from build123d import *

# Parameters (mm, degrees)
F0_W          = 12.7
F0_H          = 12.7
F1_DEPTH      = 12.7
F2_R          = 6.35
F3_DEPTH      = 12.7
F4_W          = 12.7
F4_H          = 12.7
F5_DEPTH      = 12.7
F7_DEPTH      = 6.351
F7_DEPTH_BACK = 6.351
F9_DEPTH      = 6.351
F9_DEPTH_BACK = 6.351


with BuildPart() as f1:
    # F0 (on Top) → F1 (new body)
    with BuildSketch(Plane.XY):
        Rectangle(F0_W, F0_H)
    extrude(amount=F1_DEPTH)

    # F2 (on face) → F3 (join)
    with BuildSketch(Plane.XY.offset(12.7)):
        Circle(F2_R)
    extrude(amount=F3_DEPTH)

    # F4 (on face) → F5 (join)
    with BuildSketch(Plane.XY.offset(25.4)):
        Rectangle(F4_W, F4_H)
    extrude(amount=F5_DEPTH)

    # F6 (on Front) → F7 (cut, two sides)
    with BuildSketch(Plane.XZ) as f7_sk:
        Polygon((-4.445, 25.4), (0, 38.1), (-6.35, 38.1), (-6.35, 25.4), align=None)
        Polygon((4.445, 25.4), (6.35, 25.4), (6.35, 38.1), (0, 38.1), align=None)
    extrude(amount=-F7_DEPTH, mode=Mode.SUBTRACT)
    extrude(f7_sk.sketch, amount=F7_DEPTH_BACK, mode=Mode.SUBTRACT)

    # F8 (on Right) → F9 (cut, two sides)
    with BuildSketch(Plane.YZ) as f9_sk:
        Polygon((1.4e-09, 38.1), (-6.35, 38.1), (-6.35, 25.4), (-4.4449999986, 25.4), align=None)
        Polygon((6.35, 38.1), (1.4e-09, 38.1), (4.4450000014, 25.4), (6.35, 25.4), align=None)
    extrude(amount=-F9_DEPTH, mode=Mode.SUBTRACT)
    extrude(f9_sk.sketch, amount=F9_DEPTH_BACK, mode=Mode.SUBTRACT)


solid = f1.part
Verification items for the finished model (mm, model axes). A direction names the side the tool comes from. Give positions to 0.01 mm unless a question says otherwise; leave off trailing zeros. Loops run counter-clockwise (first coordinate to the right, second up) from the corner with the lowest first, then second, coordinate; pieces in that order, holes last.
1) Sectioned sample at A-A, the plane y = -2.5. Enter the section's corners in (x, z) (3 decimals).
2) Sectioned sample at D-D, the plane z = 29. Enter the section's corners in (x, y) (3 decimals), then the cut area to 3 significant figures.
3) Sectioned sample at C-C, the plane z = 33.5. Enter the section's corners in (x, y), then the cut area to 3 significant figures.
4) Thickness scan on line 1 along Z through (x, y) = (-4.25, 6); line 2 along Z through (x, y) = (2.25, 5.5); line 3 along Y through (x, z) = (5, 15). Record the ranges inside material, lowest first.
5) Depth check by flat-ended pin: pin 1 Ø5 at (x, z) = (-1, 24) entering from +Y; pin 2 Ø5 at (x, y) = (4, -4.5) entering from +Z; pin 3 Ø5 at (x, z) = (4, 27) entering from +Y; pin 4 Ø5 at (x, y) = (-4.5, -3) entering from +Z. Enter the tip coordinate at first touch or a pass-through.
6) Set-up check for faces 1 (the flat face through (-5, -5, 12.7)), 2 (the flat face through (5, 5, 12.7)), 3 (the cylindrical face through (-1.38, -6.2, 18.96)), 4 (the flat face through (-5, 5, 12.7)), 5 (the flat face through (5, -5, 12.7)): record each of +Z, -Z, +X, -X, +Y, -Y from which the full face is reachable in a straight line by a thin tool's end or side.
7) Sectioned sample at B-B, the plane z = 24.5. Enter the section's corners in (x, y), then the cut area to 3 significant figures.
Answers:
1. outline: (-6.35, 0) - (6.35, 0) - (6.35, 12.7) - (5.837, 12.7) - (5.837, 25.4) - (4.445, 25.4) - (2.5, 30.957) - (-2.5, 30.957) - (-4.445, 25.4) - (-5.837, 25.4) - (-5.837, 12.7) - (-6.35, 12.7) - close
2. outline: (-3.185, -3.185) - (3.185, -3.185) - (3.185, 3.185) - (-3.185, 3.185) - close
2. area: 40.6 mm2
3. outline: (-1.61, -1.61) - (1.61, -1.61) - (1.61, 1.61) - (-1.61, 1.61) - close
3. area: 10.4 mm2
4. line 1: z = 0 to 12.7
4. line 2: z = 0 to 25.4
4. line 3: y = -3.91 to 3.91
5. pin 1: stops at y = 6.35
5. pin 2: stops at z = 30.96
5. pin 3: stops at y = 6
5. pin 4: stops at z = 31.96
6. face 1: +Z, -X, -Y
6. face 2: +Z, +X, +Y
6. face 3: +Z
6. face 4: +Z, -X, +Y
6. face 5: +Z, +X, -Y
7. outline: circle Ø12.7 at (0, 0)
7. area: 127 mm2
